Check sheet for the modelled part. Datum: model origin and axes. Units: mm. Give positions to 0.01 mm unless a question says otherwise; leave off trailing zeros. Loops run counter-clockwise (first coordinate to the right, second up) from the corner with the lowest first, then second, coordinate; pieces in that order, holes last.
Autodesk Inventor part; units mm, degrees
ref_plane "YZ Plane" through (0, 0, 0) normal (1, 0, 0) x (0, 1, 0)
ref_plane "XZ Plane" through (0, 0, 0) normal (0, 1, 0) x (-1, 0, 0)
ref_plane "XY Plane" through (0, 0, 0) normal (0, 0, 1) x (1, 0, 0)
sketch "スケッチ1" plane through (0, 0, 0) normal (1, 0, 0) x (0, 1, 0)
  line L0 (-105, 5) -> (105, 5)
  line L1 (105, 5) -> (105, -5)
  line L2 (105, -5) -> (-105, -5)
  line L3 (-105, -5) -> (-105, 5)
  circle A0 centre (-105, 0) radius 5
  circle A1 centre (105, 0) radius 5
  point P0 (0, 0)
  point P1 (0, 5)
  dimension "d0" = 210
  dimension "d1" = 10
  dimension "d2" = 5
  dimension "d3" = 105
extrude "押し出し1" add sketch "スケッチ1" along normal blind 5 and the other way blind 5 contours A0 L3 | L0 A1 L2 A0 | L1 A1 picked at (-103.4984, 0.7231) picked at (102.0793, -0.9468)
extrude "押し出し2" add sketch "スケッチ1" along normal blind 7.5 and the other way blind 7.5 contours A0 L3 | L3 A0 | A1 L1 | L1 A1
(1) Material ranges on line 1 (X direction, y = 44.5, z = 4.75); line 2 (Y direction, x = 6.25, z = -3.75); line 3 (Y direction, x = 0.5, z = -0.25), recorded low to high.
(2) Section check A-A on z = 3. Record the boundary of the cut face in (x, y).
(3) Gauge pin test, flat ends, axial feed: pin 1 Ø3 at (y, z) = (38.5, -1) entering from +X; pin 2 Ø4 at (x, z) = (1, 3) entering from +Y; pin 3 Ø3 at (y, z) = (-3, -2.5) entering from -X. Record the tip position at first contact, or that the pin passes through.
(4) Release check for a two-part mould opening along Y. For faces 1 (the face through (0, 1, -5)), 2 (the face through (0.105, 109.619, -1.915)) record: pulls with the +Y half, pulls with the -Y half, needs draft (parallel to the pull), parting line crosses it, or undercut.
(5) Section check B-B on y = -86. Record the boundary of the cut face in (x, z), plus the area to 3 significant figures.
Computed values:
1. line 1: x = -5 to 5
1. line 2: y = -108.31 to -101.69, 101.69 to 108.31
1. line 3: y = -109.99 to 109.99
2. outline: (-7.5, -109) - (7.5, -109) - (7.5, -101) - (5, -101) - (5, 101) - (7.5, 101) - (7.5, 109) - (-7.5, 109) - (-7.5, 101) - (-5, 101) - (-5, -101) - (-7.5, -101) - close
3. pin 1: stops at x = 5
3. pin 2: stops at y = 109.9
3. pin 3: stops at x = -5
4. face 1: needs draft
4. face 2: undercut
5. outline: (-5, -5) - (5, -5) - (5, 5) - (-5, 5) - close
5. area: 100 mm2
